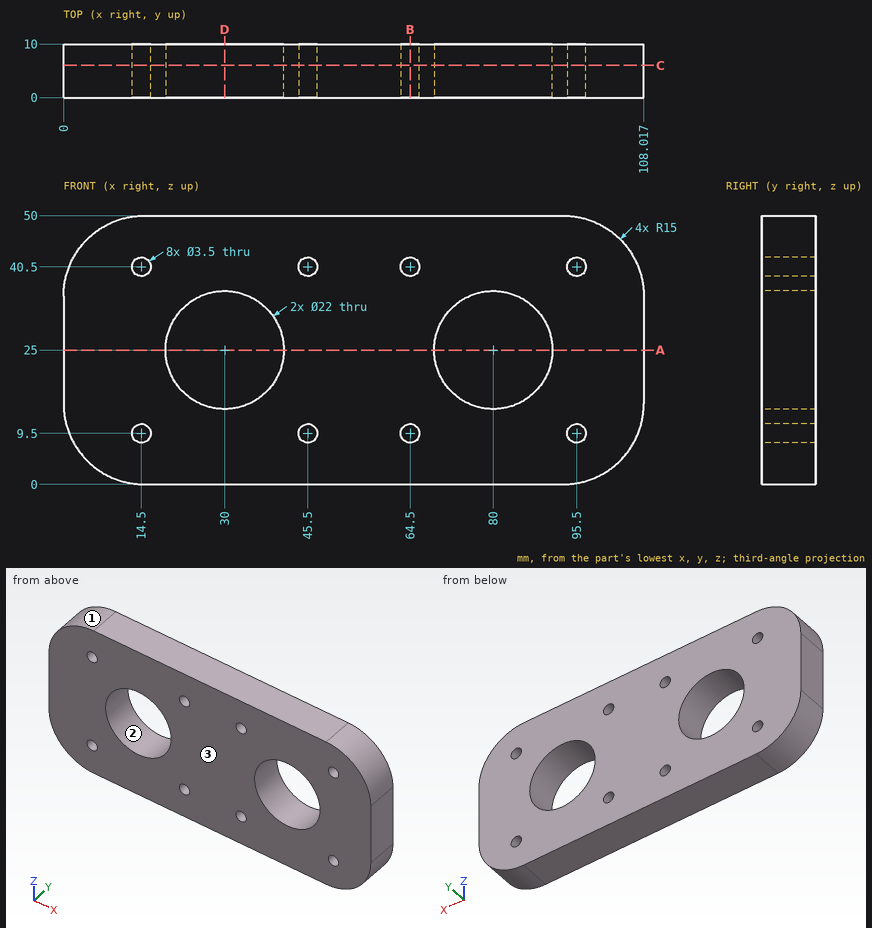
Part print with two shaded views. Sizes in mm from the minimum x, y, z corner. Round coordinates to 2 decimals unless told otherwise and drop trailing zeros. Order: outer loops, then holes, each group sorted by start corner. A loop starts at its lowest first (then second) coordinate and runs counter-clockwise, first axis right, second up. Notation, with made-up numbers: M 67,82.5 L 72,82.5 A27 ccw 72,109.5 Z; hole C 58,21.5 d1. An arc over 180 degrees is marked long. Put each result on its own line as item: value. Start each with the question number.
1. Slice it at D-D on x = 30. List the corners of the cut face in (y, z).
2. Drill centre lines: probe 1 along Z at (x, y) = (64.5, 6); probe 2 along Z at (x, y) = (16, 9); probe 3 along X at (y, z) = (6.5, 17). Where is each one in solid material? Low to high. Write a range as [from, to].
3. Drop a flat-ended pin along its axis: pin 1 (4.5 mm diameter, centred on x = 64.5, z = 40.5, fed in from +Y). Give the stop position or say it passes through.
4. Slice it at A-A on z = 25. List the corners of the cut face in (x, y), then the cut area to 3 significant figures.
5. Slice it at B-B on x = 64.5. List the corners of the cut face in (y, z).
6. Two-plate mould, pull along X, no slides. Class the marked faces 1, 2 and 3: +X half, -X half, draft (parallel to the pull), parting line (faces both ways), or undercut.
7. Slice it at C-C on y = 6. State how many separate pieces and enclosed holes the cut face has, then the cut area to 3 significant figures.
Findings:
1. outline: M 0,0 L 10,0 L 10,14 L 0,14 Z; M 0,36 L 10,36 L 10,50 L 0,50 Z
2. probe 1: [0, 7.75], [11.25, 38.75], [42.25, 50]
2. probe 2: [0, 8.6], [10.4, 39.6], [41.4, 50]
2. probe 3: [0, 22.45], [37.55, 72.45], [87.55, 108.02]
3. pin 1: y = 10
4. outline: M 0,0 L 19,0 L 19,10 L 0,10 Z; M 41,0 L 69,0 L 69,10 L 41,10 Z; M 91,0 L 108.02,0 L 108.02,10 L 91,10 Z
4. area: 640 mm2
5. outline: M 0,0 L 10,0 L 10,7.75 L 0,7.75 Z; M 0,11.25 L 10,11.25 L 10,38.75 L 0,38.75 Z; M 0,42.25 L 10,42.25 L 10,50 L 0,50 Z
6. face 1: -X half
6. face 2: undercut
6. face 3: draft
7. separate pieces: 1
7. enclosed holes: 10
7. area: 4,370 mm2
